```python
from build123d import *

# Parameters (mm, degrees)
F1_DEPTH = 25
F2_T     = -2.5


with BuildPart() as f1:
    # F0 (on Front) → F1 (new body, symmetric)
    with BuildSketch(Plane.XZ):
        Polygon((33.765722, 23.008151), (-33.244941, 23.008151), (-33.244941, -13.642579), (-13.2785, -13.642579), (-13.2785, 0), (12.431712, 0), (12.431712, -13.642579), (33.765722, -13.642579), align=None)
    extrude(amount=F1_DEPTH, both=True)

    # F2
    f2_openings = [f1.faces().sort_by_distance(p)[0] for p in [
        (-0.423394, 0, 0),
        (23.098717, 0, -13.642579),
        (-23.261721, 0, -13.642579),
        (-13.2785, 0, -6.82129),
        (12.431712, 0, -6.82129),
    ]]
    offset(amount=F2_T, openings=f2_openings)


solid = f1.part
```
Input: part model. Units: mm. Frame: model coordinates. A direction names the side the tool comes from. Coordinates: 2 decimals unless noted, no trailing zeros. Loops run counter-clockwise (first coordinate to the right, second up) from the corner with the lowest first, then second, coordinate; pieces in that order, holes last. Notation, with made-up numbers: M 8,68.25 L 53,68.25 A19 cw 53,105.25 Z; hole C -27.75,85 d11. An arc over 180 degrees is marked long. Answer in a Markdown table with one row per item.
1. Section A-A, the plane z = -8. Output: boundary loops of the cut face in (x, y).
Response:
| item | result |
|---|---|
| outline | M -33.24,-25 L -13.28,-25 L -13.28,-22.5 L -30.74,-22.5 L -30.74,22.5 L -13.28,22.5 L -13.28,25 L -33.24,25 Z; M 12.43,-25 L 33.77,-25 L 33.77,25 L 12.43,25 L 12.43,22.5 L 31.27,22.5 L 31.27,-22.5 L 12.43,-22.5 Z |
2. Section B-B, the plane x = -15.5. Output: boundary loops of the cut face in (y, z), then the cut area to 3 significant figures.
Response:
| item | result |
|---|---|
| outline | M -25,-13.64 L -22.5,-13.64 L -22.5,20.51 L 22.5,20.51 L 22.5,-13.64 L 25,-13.64 L 25,23.01 L -25,23.01 Z |
| area | 296 mm2 |
3. Section C-C, the plane z = 2.5. Output: boundary loops of the cut face in (x, y), then the cut area to 3 significant figures.
Response:
| item | result |
|---|---|
| outline | M -33.24,-25 L 33.77,-25 L 33.77,25 L -33.24,25 Z; hole M -30.74,-22.5 L 31.27,-22.5 L 31.27,22.5 L -30.74,22.5 Z |
| area | 560 mm2 |
4. Material intervals for line 1 (X direction, y = -8.5, z = 17.5); line 2 (Y direction, x = -2.5, z = 16.5); line 3 (Z direction, x = 5, y = -22), sorted ascending.
Response:
| item | result |
|---|---|
| line 1 | x = -33.24 to -30.74, 31.27 to 33.77 |
| line 2 | y = -25 to -22.5, 22.5 to 25 |
| line 3 | z = 20.51 to 23.01 |
5. Section D-D, the plane y = 15.5. Output: boundary loops of the cut face in (x, z), then the cut area to 3 significant figures.
Response:
| item | result |
|---|---|
| outline | M -33.24,-13.64 L -30.74,-13.64 L -30.74,20.51 L 31.27,20.51 L 31.27,-13.64 L 33.77,-13.64 L 33.77,23.01 L -33.24,23.01 Z |
| area | 338 mm2 |
6. Draft query along Y for faces 4 (the flat face through (0, -25, 5)), 5 (the flat face through (0, 25, 5)), 6 (the flat face through (1, 0, 23.008)), 7 (the flat face through (-30.745, 0, 4)). Return one class per face: pulls with the +Y half, pulls with the -Y half, needs draft (parallel to the pull), parting line crosses it, or undercut.
Response:
| item | result |
|---|---|
| face 4 | pulls with the -Y half |
| face 5 | pulls with the +Y half |
| face 6 | needs draft |
| face 7 | undercut |
7. Reachability of faces 1 (the flat face through (31.266, 0, 3)), 2 (the flat face through (-31, 0, -13.643)), 3 (the flat face through (-1, -24, 0)) from +Z, -Z, +X, -X, +Y, -Y: full face, straight path, thin tool, end or side. Return the list, or none.
Response:
| item | result |
|---|---|
| face 1 | -Z |
| face 2 | -Z, +X, -X, +Y, -Y |
| face 3 | -Z, +Y, -Y |
8. First-contact query: pin 1 (2 mm diameter, centred on x = 17.5, y = -17.5, fed in from -Z); pin 2 (3 mm diameter, centred on x = 1.5, y = 24, fed in from -Z). Flat tips, straight axial feed; report the tip coordinate or a pass-through.
Response:
| item | result |
|---|---|
| pin 1 | stops at z = 20.51 |
| pin 2 | stops at z = 0 |
